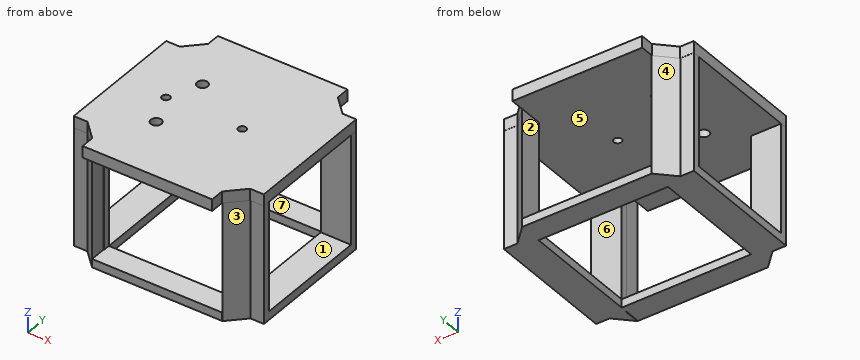
Autodesk Inventor part; units mm, degrees
ref_plane "Work Plane1" through (-56.3599, 0, 22) normal (0, 0, -1) x (-1, 0, 0)
ref_plane "Arbeitsebene9" through (-61.2799, 5.9299, 18.95) normal (0, 0, 1) x (1, 0, 0)
ref_plane "Arbeitsebene10" through (-18.4599, -3.9201, -16.28) normal (-1, 0, 0) x (0, 0, 1)
ref_plane "Work Plane1" through (-56.3599, 0, 22) normal (0, 0, -1) x (-1, 0, 0)
ref_plane "Arbeitsebene9" through (-61.2799, 5.9299, 18.95) normal (0, 0, 1) x (1, 0, 0)
sketch "Sketch1" plane through (-56.3599, 0, 22) normal (0, 0, -1) x (-1, 0, 0)
  line L0 (-4.0299, -0.3538) -> (-2.2322, 1.4439) construction
  arc A0 (-1.4439, 2.2322) -> (-2.2322, 1.4439) centre (-0.9299, 0.9299) ccw construction
  line L1 (-1.4439, 2.2322) -> (0.3538, 4.0299) construction
  line L2 (-37.8299, 42.8299) -> (-37.8299, 37.8299) construction
  line L3 (-37.8299, 37.8299) -> (-42.9208, 37.8299) construction
  line L4 (-37.8299, 42.2137) -> (-37.8299, 45.8299) construction
  line L5 (-37.8299, 45.8299) -> (-4.0299, 45.8299) construction
  line L6 (-4.0299, 45.8299) -> (-4.0299, 42.2137) construction
  line L7 (-4.0299, 4.0299) -> (0.3538, 4.0299)
  circle A1 centre (-20.9299, 20.9299) radius 17.5
  line L8 (-20.9299, 58.9723) -> (17.1124, 20.9299) construction
  line L9 (17.1124, 20.9299) -> (-20.9299, -17.1124) construction
  line L10 (-20.9299, -17.1124) -> (-58.9723, 20.9299) construction
  line L11 (-58.9723, 20.9299) -> (-20.9299, 58.9723) construction
  line L12 (-20.9299, 58.9723) -> (-20.9299, -17.1124) construction
  line L13 (17.1124, 20.9299) -> (-58.9723, 20.9299) construction
  line L14 (-20.9299, 58.9723) -> (32.8701, 58.9723) construction
  line L15 (-43.4299, 43.4299) -> (1.5701, 43.4299) construction
  line L16 (1.5701, 43.4299) -> (1.5701, -1.5701) construction
  line L17 (1.5701, -1.5701) -> (-43.4299, -1.5701) construction
  line L18 (-43.4299, -1.5701) -> (-43.4299, 43.4299) construction
  line L19 (-43.4299, 43.4299) -> (1.5701, -1.5701) construction
  line L20 (1.5701, 43.4299) -> (-43.4299, -1.5701) construction
  line L21 (-43.4299, 5.3876) -> (-43.4299, 36.4723)
  line L22 (-43.4299, 36.4723) -> (-36.4723, 43.4299)
  line L23 (-36.4723, 43.4299) -> (-5.3876, 43.4299)
  line L24 (-5.3876, 43.4299) -> (1.5701, 36.4723)
  line L25 (1.5701, 36.4723) -> (1.5701, 5.3876)
  line L26 (1.5701, 5.3876) -> (-5.3876, -1.5701)
  line L27 (-5.3876, -1.5701) -> (-36.4723, -1.5701)
  line L28 (-36.4723, -1.5701) -> (-43.4299, 5.3876)
  line L29 (-4.0299, 42.2137) -> (-37.8299, 42.2137)
  line L30 (-4.0299, -0.3538) -> (-4.0299, 4.0299)
  circle A2 centre (-20.9299, 20.9299) radius 1.5
  line L31 (-10.9299, 10.9299) -> (-30.9299, 10.9299) construction
  line L32 (-30.9299, 10.9299) -> (-30.9299, 30.9299) construction
  line L33 (-30.9299, 30.9299) -> (-10.9299, 30.9299) construction
  line L34 (-10.9299, 30.9299) -> (-10.9299, 10.9299) construction
  line L35 (-10.9299, 10.9299) -> (-30.9299, 30.9299) construction
  line L36 (-30.9299, 10.9299) -> (-10.9299, 30.9299) construction
  circle A3 centre (-30.9299, 30.9299) radius 1.4
  circle A4 centre (-30.9299, 10.9299) radius 1.4
  circle A5 centre (-10.9299, 10.9299) radius 1.4
  line L37 (-45.8299, 37.8299) -> (-42.0723, 37.8299) construction
  line L38 (-42.1723, 37.7299) -> (-45.8299, 37.7299)
  line L39 (-45.8299, 37.7299) -> (-45.8299, 4.1299)
  line L40 (-45.8299, 4.1299) -> (-42.1723, 4.1299)
  line L41 (-42.1723, 4.1299) -> (-42.1723, 37.7299)
  line L42 (-45.8299, 4.0299) -> (-42.0723, 4.0299) construction
  line L43 (-45.8299, 37.8299) -> (-42.0723, 37.8299)
  line L44 (-37.7299, 45.8299) -> (-4.1299, 45.8299)
  line L45 (-4.1299, 45.8299) -> (-4.1299, 42.1723)
  line L46 (-4.1299, 42.1723) -> (-37.7299, 42.1723)
  line L47 (-37.7299, 42.1723) -> (-37.7299, 45.8299)
  line L48 (0.4701, 37.8299) -> (0.4701, 4.0299) construction
  line L49 (0.4701, 4.0299) -> (3.9701, 4.0299) construction
  line L50 (3.9701, 37.8299) -> (3.9701, 4.0299) construction
  line L51 (0.4701, 37.8299) -> (3.9701, 37.8299) construction
  line L52 (-45.8299, -3.9701) -> (-4.0299, -3.9701) construction
  line L53 (0.3124, 37.7299) -> (3.9701, 37.7299)
  line L54 (3.9701, 37.7299) -> (3.9701, 4.1299)
  line L55 (3.9701, 4.1299) -> (0.3124, 4.1299)
  line L56 (0.3124, 4.1299) -> (0.3124, 37.7299)
  line L57 (-4.1713, -0.3538) -> (-37.7299, -0.3538)
  line L58 (-37.7299, -0.3538) -> (-37.7299, -3.9701)
  line L59 (-37.7299, -3.9701) -> (-4.1713, -3.9701)
  line L60 (-4.1713, -3.9701) -> (-4.1713, -0.3538)
  point P0 (-37.8299, 4.0299)
  dimension "d18" = 53.8
  dimension "d19" = 45
  dimension "d20" = 53.8
  dimension "d21" = 45
  dimension "d22" = 45
  dimension "d30" = 20
  dimension "d31" = 20
  dimension "d32" = 2.8
  dimension "d33" = 2.8
  dimension "d34" = 2.8
  dimension "d35" = 3
  dimension "d36" = 0.1
  dimension "d37" = 0.1
  dimension "d38" = 0.1
  dimension "d39" = 0.1
extrude "Extrusion1" add sketch "Sketch1" along normal up to surface (3.05 mm away) contours L30 L26 L57 L28 L41 L22 L46 L24 L56 L7 | L7 L26 L30 | L56 L24 L25 L26 | L26 L25 L24 L53 L54 L55 | L60 L59 L58 L57 L28 L27 L26 | L26 L27 L28 L57 | L46 L22 L29 L24 | L24 L29 L45 | L40 L39 L38 L22 L21 L28 | L28 L21 L22 L41 | L29 L22 L23 L24 | L24 L23 L22 L29 L47 L44 L45 | L47 L29 L22 | A1 | A2 | A3 | A4 | A5
sketch "Skizze4" plane through (-56.3599, 0, 18.95) normal (0, 0, -1) x (-1, 0, 0)
  line L0 (-37.7299, 42.1723) -> (-42.1723, 37.7299)
  line L1 (-42.1723, 37.7299) -> (-45.8299, 37.7299)
  line L2 (-45.8299, 37.7299) -> (-45.8299, 4.1299) construction
  line L3 (-45.8299, 4.1299) -> (-42.1723, 4.1299)
  line L4 (-42.1723, 4.1299) -> (-37.6885, -0.3538)
  line L5 (-37.6885, -0.3538) -> (-37.7299, -0.3538)
  line L6 (-37.7299, -0.3538) -> (-37.7299, -3.9701)
  line L7 (-37.7299, -3.9701) -> (-4.1713, -3.9701) construction
  line L8 (-4.1713, -3.9701) -> (-4.1713, -0.3538)
  line L9 (-4.1713, -0.3538) -> (0.3124, 4.1299)
  line L10 (0.3124, 4.1299) -> (3.9701, 4.1299)
  line L11 (3.9701, 4.1299) -> (3.9701, 37.7299) construction
  line L12 (3.9701, 37.7299) -> (0.3124, 37.7299)
  line L13 (0.3124, 37.7299) -> (-4.1299, 42.1723)
  line L14 (-4.1299, 42.1723) -> (-4.1299, 45.8299)
  line L15 (-4.1299, 45.8299) -> (-37.7299, 45.8299) construction
  line L16 (-37.7299, 45.8299) -> (-37.7299, 42.1723)
  line L17 (-37.9299, 46.0299) -> (-3.9299, 46.0299) construction
  line L18 (-3.9299, 46.0299) -> (-3.9299, 42.2551)
  line L19 (-3.9299, 42.2551) -> (0.3953, 37.9299)
  line L20 (0.3953, 37.9299) -> (4.1701, 37.9299)
  line L21 (4.1701, 37.9299) -> (4.1701, 3.9299) construction
  line L22 (4.1701, 3.9299) -> (0.3953, 3.9299)
  line L23 (0.3953, 3.9299) -> (-3.9713, -0.4367)
  line L24 (-3.9713, -0.4367) -> (-3.9713, -4.1701)
  line L25 (-3.9713, -4.1701) -> (-37.9299, -4.1701) construction
  line L26 (-37.9299, -4.1701) -> (-37.9299, -0.3953)
  line L27 (-37.9299, -0.3953) -> (-42.2551, 3.9299)
  line L28 (-42.2551, 3.9299) -> (-46.0299, 3.9299)
  line L29 (-46.0299, 3.9299) -> (-46.0299, 37.9299) construction
  line L30 (-46.0299, 37.9299) -> (-42.2551, 37.9299)
  line L31 (-42.2551, 37.9299) -> (-37.9299, 42.2551)
  line L32 (-37.9299, 42.2551) -> (-37.9299, 46.0299)
  line L33 (-45.8299, 37.7299) -> (-45.8299, 37.9299)
  line L34 (-4.1299, 45.8299) -> (-37.7299, 45.8299)
  line L35 (-37.7299, 45.8299) -> (-37.9299, 45.8299)
  line L36 (-4.1299, 45.8299) -> (-3.9299, 45.8299)
  line L37 (3.9701, 37.7299) -> (3.9701, 37.9299)
  line L38 (3.9701, 4.1299) -> (3.9701, 37.7299)
  line L39 (3.9701, 4.1299) -> (3.9701, 3.9299)
  line L40 (-4.1713, -3.9701) -> (-3.9713, -3.9701)
  line L41 (-37.7299, -3.9701) -> (-37.9299, -3.9701)
  line L42 (-45.8299, 4.1299) -> (-45.8299, 3.9299)
  point P0 (-56.3599, 0)
  dimension "d40" = 0.2
extrude "IM_offset" add sketch "Skizze4" against normal up to surface (3.05 mm away)
ref_plane "Arbeitsebene5" through (-35.4299, 3.9299, 22) normal (-1, 0, 0) x (0, 0, 1)
ref_plane "Arbeitsebene6" through (-18.4299, 20.9299, 22) normal (0, 1, 0) x (-1, 0, 0)
sketch "Skizze31" plane through (-10.5299, 3.9299, 18.95) normal (1, 0, 0) x (0, 0, -1)
  line L0 (0, 0) -> (0, 34)
  line L1 (0, 34) -> (-3.05, 34)
  line L2 (-3.05, 0) -> (-3.05, 34)
  line L3 (0, 0) -> (-3.05, 0)
  line L4 (-3.05, -5.85) -> (-10.55, -5.85)
  line L5 (-3.05, 33.97) -> (-3.05, -5.85)
  line L6 (-3.05, 33.97) -> (31.05, 33.97)
  line L7 (31.05, 39.85) -> (31.05, 33.97)
  line L8 (-10.55, 39.85) -> (31.05, 39.85)
  line L9 (-10.55, -5.85) -> (-10.55, 39.85)
  line L10 (31.05, 39.85) -> (38.55, 39.85)
  line L11 (31.05, 0.03) -> (31.05, 39.85)
  line L12 (31.05, 0.03) -> (-3.05, 0.03)
  line L13 (-3.05, -5.85) -> (-3.05, 0.03)
  line L14 (38.55, -5.85) -> (-3.05, -5.85)
  line L15 (38.55, 39.85) -> (38.55, -5.85)
  line L16 (0, 0) -> (0, 34)
  line L17 (0, 33.97) -> (30.9, 33.97)
  line L18 (30.9, 33.97) -> (30.9, 32.1075)
  line L19 (30.9, 32.1075) -> (0, 32.1075)
  line L20 (0, 32.1075) -> (0, 33.97)
  line L21 (30.9, 1.8846) -> (0, 1.8846)
  line L22 (0, 1.8846) -> (0, 0.03)
  line L23 (0, 0.03) -> (30.9, 0.03)
  line L24 (30.9, 0.03) -> (30.9, 1.8846)
  circle A0 centre (20.35, 17) radius 6.5
  line L25 (30.9, 32.1075) -> (30.9, 1.8846)
  line L26 (28.5, 2) -> (28.5, 32)
  line L27 (28.7, 32.1075) -> (28.7, 1.8846)
  point P0 (18.95, -3.9299)
  point P1 (0, 33.97)
  point P2 (0, 1.8846)
  point P3 (0, 0.03)
  dimension "d181" = 0
  dimension "d182" = 0
  dimension "d183" = 0.15
  dimension "d184" = 0.2
ref_plane "Arbeitsebene10" through (-18.4599, -3.9201, -16.28) normal (-1, 0, 0) x (0, 0, 1)
extrude "Extrusion26" add sketch "Skizze31" against normal up to surface (7.93 mm away) contours L0 L21 L24 L12 | L0 L6 L18 L19 | L27 L19 L25 L21
sketch "Skizze32" plane through (-10.5299, 3.9599, -11.95) normal (0, 0, -1) x (-1, 0, 0)
  line L0 (0, 0) -> (0, 33.94)
  line L1 (0, 33.94) -> (7.93, 33.94)
  line L2 (0, 0) -> (7.93, 0)
  line L3 (7.9, -4.3552) -> (3.5748, -0.03) construction
  line L4 (4.3761, 34.7834) -> (7.1197, 37.7973) construction
  line L5 (7.9, 38.2952) -> (3.5748, 33.97) construction
  line L6 (3.5448, 33.94) -> (7.93, 38.3252)
  line L7 (7.93, 38.3252) -> (7.93, 33.94)
  line L8 (7.93, 1.8546) -> (7.93, 0)
  line L9 (7.93, 0) -> (7.93, -0.13)
  line L10 (3.5448, 0) -> (7.8, -4.2552)
  line L11 (7.8, -4.2552) -> (7.8, 0)
  point P0 (-10.5299, -3.9599)
  dimension "d187" = 45
  dimension "d188" = 0
  dimension "d189" = 0
extrude "Extrusion27" add sketch "Skizze32" against normal up to surface (30.9 mm away)
mirror "Spiegeln2" about plane through (-35.4299, 3.9299, 22) normal (-1, 0, 0) of "Extrusion26", "Extrusion27"
sketch "Skizze33" plane through (-10.5299, 3.9599, -11.95) normal (0, 0, -1) x (-1, 0, 0)
  line L0 (0.05, 39.82) -> (0.05, -5.88)
  line L1 (41.87, 0) -> (41.87, 38.3252)
  line L2 (7.93, 0) -> (7.93, 38.3252)
  line L3 (41.87, 38.3252) -> (7.93, 38.3252)
  line L4 (7.93, 38.3252) -> (7.93, 32.3252)
  line L5 (7.93, 32.3252) -> (41.87, 32.3252)
  line L6 (41.87, 32.3252) -> (41.87, 38.3252)
  line L7 (46.2552, 0) -> (42, -4.2552)
  line L8 (42, -4.2552) -> (7.93, -4.2552)
  line L9 (7.93, -4.2552) -> (7.93, 1.7448)
  line L10 (7.93, 1.7448) -> (42, 1.7448)
  line L11 (42, 1.7448) -> (42, -4.2552)
  point P0 (-10.5299, -3.9599)
  point P1 (7.93, 38.3252)
  point P2 (41.87, 32.3252)
  dimension "d192" = 6
  dimension "d193" = 6
extrude "Extrusion28" add sketch "Skizze33" against normal up to surface (2.2 mm away) contours L5 L2 L3 L1 | L10 L11 L8 L9 L2
sketch "Skizze34" plane through (-56.3599, 0, 22) normal (0, 0, 1) x (1, 0, 0)
  line L0 (-4.9201, 35.9299) -> (-4.9201, 5.9299)
  line L1 (83.0799, 5.9299) -> (-4.9201, 5.9299)
  line L2 (83.0799, 35.9299) -> (83.0799, 5.9299)
  line L3 (83.0799, 35.9299) -> (-4.9201, 35.9299)
  circle A0 centre (8.0799, 20.9299) radius 1.025
  circle A1 centre (28.0799, 20.9299) radius 1.025
  circle A2 centre (48.0799, 20.9299) radius 1.025
  circle A3 centre (68.0799, 20.9299) radius 1.025
  circle A4 centre (66.5799, 29.4299) radius 1.7
  circle A5 centre (66.5799, 12.4299) radius 1.7
  circle A6 centre (11.5799, 12.4299) radius 1.7 construction
  circle A7 centre (11.5799, 29.4299) radius 1.7 construction
  circle A8 centre (11.5799, 12.4299) radius 1.4
  circle A9 centre (11.5799, 29.4299) radius 1.4
  point P0 (56.3599, 0)
  dimension "d198" = 2.8
  dimension "d199" = 2.8
extrude "Extrusion29" cut sketch "Skizze34" against normal blind 10 contours A0 | A1 | A8 | A9
properties part number "20_Cube_Insert_Cube_Z-Stage_NEMA11_china_v3"
Part model, mm, in its own coordinate system. Face numbers are marked on the shaded views. A direction names the side the tool comes from. Coordinates: 2 decimals unless noted, no trailing zeros. Write each loop counter-clockwise with the first axis right and the second up, starting at its lowest first coordinate (ties: lowest second). Pieces come first, ordered by that corner, then holes. Notation, with made-up numbers: (16, 39) - (75, 39) arc R33 cw to (75, 76) - close; hole circle Ø4 at (55.25, 33.25). An arc over 180 degrees is marked (long way). Put each result on its own line as item: value.
1. Probe line 1 along Y through (x, z) = (-44.78, 20.15); line 2 along Y through (x, z) = (-48.28, 20.8); line 3 along Y through (x, z) = (-44, 19). List the from-to ranges inside material, lowest first. Write a range as [from, to].
Final values:
line 1: y = [-3.97, 11.03], [13.83, 28.03], [30.83, 45.83]
line 2: y = [-3.97, 19.9], [21.95, 45.83]
line 3: y = [-3.97, 11.27], [13.59, 28.27], [30.59, 45.83]
2. Two-plate mould, pull along Y, no slides. Class the marked faces 4, 5, 6 and 7: +Y half, -Y half, draft (parallel to the pull), parting line (faces both ways), or undercut.
Final values:
face 4: +Y half
face 5: undercut
face 6: undercut
face 7: draft
3. Band-saw the part on D-D (x = -39.5). Write the cut outline in (y, z).
Final values:
outline: (-3.97, 18.95) - (45.83, 18.95) - (45.83, 22) - (-3.97, 22) - close; (-0.3, -11.95) - (5.7, -11.95) - (5.7, -9.75) - (-0.3, -9.75) - close; (36.29, -11.95) - (42.29, -11.95) - (42.29, -9.75) - (36.29, -9.75) - close
4. Band-saw the part on C-C (x = -28.28). Write the cut outline in (y, z).
Final values:
outline: (-3.97, 18.95) - (19.9, 18.95) - (19.9, 22) - (-3.97, 22) - close; (-0.3, -11.95) - (5.7, -11.95) - (5.7, -9.75) - (-0.3, -9.75) - close; (21.95, 18.95) - (45.83, 18.95) - (45.83, 22) - (21.95, 22) - close; (36.29, -11.95) - (42.29, -11.95) - (42.29, -9.75) - (36.29, -9.75) - close
5. Band-saw the part on B-B (y = 25.5). Write the cut outline in (x, z).
Final values:
outline: (-60.33, -11.95) - (-52.4, -11.95) - (-52.4, -9.75) - (-60.33, -9.75) - close; (-60.33, 18.95) - (-10.53, 18.95) - (-10.53, 22) - (-60.33, 22) - close; (-18.46, -11.95) - (-10.53, -11.95) - (-10.53, -9.75) - (-18.46, -9.75) - close
6. Band-saw the part on A-A (z = 7). Write the cut outline in (x, y).
Final values:
outline: (-60.33, 3.96) - (-56.79, 3.96) - (-52.53, -0.3) - (-52.53, 3.96) - (-52.4, 3.96) - (-52.4, 5.81) - (-60.33, 5.81) - close; (-60.33, 36.04) - (-52.4, 36.04) - (-52.4, 42.29) - (-56.79, 37.9) - (-60.33, 37.9) - close; (-18.46, 3.96) - (-18.33, 3.96) - (-18.33, -0.3) - (-14.07, 3.96) - (-10.53, 3.96) - (-10.53, 5.81) - (-18.46, 5.81) - close; (-18.46, 36.04) - (-10.53, 36.04) - (-10.53, 37.9) - (-14.07, 37.9) - (-18.46, 42.29) - close
7. 3-axis set-ups, long thin cutter, end or side, ignore diameter. For the marked faces 1, 2 and 3: which of +Z, -Z, +X, -X, +Y, -Y reach the whole face in a straight line?
Final values:
face 1: +X, -X
face 2: none
face 3: +Z, -Z, +X, -Y
8. Flat gauge pins, fed straight in: pin 1 Ø1.5 at (y, z) = (-2.5, 21) entering from -X; pin 2 Ø3 at (x, z) = (-16.5, 7) entering from -Y; pin 3 Ø12 at (x, y) = (-43, 22) entering from -Z; pin 4 Ø8 at (y, z) = (12, 1) entering from -X. Where does each tip first touch, or does it go through?
Final values:
pin 1: stops at x = -52.39
pin 2: stops at y = 0.03
pin 3: stops at z = 18.95
pin 4: passes through
